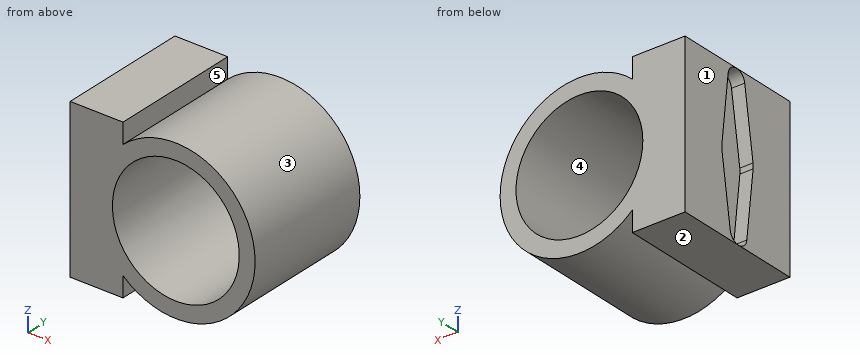
Autodesk Inventor part; units mm, degrees
ref_plane "YZ Plane" through (0, 0, 0) normal (1, 0, 0) x (0, 1, 0)
ref_plane "XZ Plane" through (0, 0, 0) normal (0, 1, 0) x (-1, 0, 0)
ref_plane "XY Plane" through (0, 0, 0) normal (0, 0, 1) x (1, 0, 0)
sketch "Sketch1" plane through (0, 0, 0) normal (0, 1, 0) x (-1, 0, 0)
  arc A0 (12, 9) -> (10, -11.1803) centre (0, 0) ccw
  line L0 (10, 15) -> (20, 15)
  line L1 (20, 15) -> (20, -15)
  line L2 (20, -15) -> (10, -15)
  line L3 (10, 15) -> (20, -15) construction
  line L4 (20, 15) -> (10, -15) construction
  line L5 (10, -15) -> (10, -11.1803)
  line L6 (10, 11.1803) -> (10, 15)
  circle A1 centre (0, 0) radius 12
  dimension "d0" = 30
  dimension "d1" = 10
  dimension "d2" = 30
  dimension "d3" = 18.435
  dimension "d4" = 20
  dimension "d5" = 24
extrude "Extrusion1" add sketch "Sketch1" along normal mid plane 25
sketch "Sketch2" plane through (-20, -12.5, 15) normal (-1, 0, 0) x (0, 0, 1)
  arc A0 (-1.6928, 10.7737) -> (-1.769, 14.7366) centre (-2, 12.75) ccw
  arc A1 (-28.3059, 14.235) -> (-28.2323, 10.2721) centre (-28, 12.2586) ccw
  line L0 (-28.3059, 14.235) -> (-15.5736, 16.2059)
  line L1 (-28.2323, 10.2721) -> (-15.4356, 8.7754)
  line L2 (-14.5668, 16.2249) -> (-1.769, 14.7366)
  line L3 (-14.4239, 8.7945) -> (-1.6928, 10.7737)
  arc A2 (-15.4356, 8.7754) -> (-14.4239, 8.7945) centre (-15, 12.5) ccw
  arc A3 (-14.5668, 16.2249) -> (-15.5736, 16.2059) centre (-15, 12.5) ccw
  dimension "d8" = 4
  dimension "d9" = 4
  dimension "d11" = 26
  dimension "d12" = 13
extrude "Extrusion2" cut sketch "Sketch2" against normal blind 2.5
properties part number "motor mount"
Geometry: final body of the model. Coordinates: model frame, mm. Face numbers are marked on the shaded views. A direction names the side the tool comes from. Round coordinates to 2 decimals unless told otherwise and drop trailing zeros. Loops run counter-clockwise (first coordinate to the right, second up) from the corner with the lowest first, then second, coordinate; pieces in that order, holes last.
Item 1: Contact query for flat-ended pins moving along their axis: P1, Ø8, axis at y = -4, z = 7, coming from the +X side; P2, Ø1, axis at y = 8.5, z = -11.5, coming from the +X side; P3, Ø4, axis at y = 2.5, z = 12.5, coming from the +X side; P4, Ø5, axis at x = -1, z = -8.5, coming from the -Y side. Output: stop coordinate, or through.
Checked values:
P1: stops at x = 14.7
P2: stops at x = 10.2
P3: stops at x = 10.71
P4: passes through
Item 2: Section A-A, the plane z = 0. Output: boundary loops of the cut face in (x, y).
Checked values:
outline: (-20, -12.5) - (-12, -12.5) - (-12, 12.5) - (-20, 12.5) - (-20, 3.75) - (-17.5, 3.75) - (-17.5, -3.75) - (-20, -3.75) - close; (12, -12.5) - (15, -12.5) - (15, 12.5) - (12, 12.5) - close
Item 3: Mould query, pull axis X, two halves, no side actions, for the marked faces 1, 2 and 3. Classes: released by +X, released by -X, zero draft, split by the parting line, or undercut.
Checked values:
face 1: released by -X
face 2: zero draft
face 3: undercut
Item 4: Section C-C, the plane y = 6. Output: boundary loops of the cut face in (x, z), plus the area to 3 significant figures.
Checked values:
outline: (-20, -15) - (-10, -15) - (-10, -11.18) arc R15 ccw (long way) to (-10, 11.18) - (-10, 15) - (-20, 15) - close; hole circle Ø24 at (0, 0)
area: 477 mm2
Item 5: Section D-D, the plane x = -4. Output: boundary loops of the cut face in (y, z), plus the area to 3 significant figures.
Checked values:
outline: (-12.5, -14.46) - (12.5, -14.46) - (12.5, -11.31) - (-12.5, -11.31) - close; (-12.5, 11.31) - (12.5, 11.31) - (12.5, 14.46) - (-12.5, 14.46) - close
area: 157 mm2
Item 6: Section B-B, the plane x = 1. Output: boundary loops of the cut face in (y, z), plus the area to 3 significant figures.
Checked values:
outline: (-12.5, -14.97) - (12.5, -14.97) - (12.5, -11.96) - (-12.5, -11.96) - close; (-12.5, 11.96) - (12.5, 11.96) - (12.5, 14.97) - (-12.5, 14.97) - close
area: 150 mm2
Item 7: Reachability of the marked faces 4 and 5 from +Z, -Z, +X, -X, +Y, -Y: full face, straight path, thin tool, end or side. Return the list, or none.
Checked values:
face 4: +Y, -Y
face 5: +Z, +Y, -Y
Item 8: Line query: L1, parallel to Z at x = 0, y = 1; L2, parallel to Z at x = -6, y = 1.25; L3, parallel to X at y = 10, z = 10. Output: solid intervals per line, ascending.
Checked values:
L1: z = -15 to -12, 12 to 15
L2: z = -13.75 to -10.39, 10.39 to 13.75
L3: x = -20 to -6.63, 6.63 to 11.18
